```python
from build123d import *

# Parameters (mm, degrees)
CLAMP_OUTLINE_SKETCH_W = 7
CLAMP_OUTLINE_SKETCH_H = 6
CLAMP_OUTLINE_DEPTH    = 1
M2_CLEARANCE_SKETCH_R  = 1.1
M2_CLEARANCE_DEPTH     = 1.2


with BuildPart() as part:
    # Clamp Outline Sketch → Clamp Outline (new body)
    with BuildSketch(Plane.XY):
        Rectangle(CLAMP_OUTLINE_SKETCH_W, CLAMP_OUTLINE_SKETCH_H)
    extrude(amount=CLAMP_OUTLINE_DEPTH)

    # M2 Clearance Sketch → M2 Clearance (cut)
    with BuildSketch(Plane.XY.offset(-0.1)):
        Circle(M2_CLEARANCE_SKETCH_R)
    extrude(amount=M2_CLEARANCE_DEPTH, mode=Mode.SUBTRACT)


solid = part.part
```
Build history of the part. All positions in model axes, mm. Round coordinates to 2 decimals unless told otherwise and drop trailing zeros. Write each loop counter-clockwise with the first axis right and the second up, starting at its lowest first coordinate (ties: lowest second). Pieces come first, ordered by that corner, then holes.
1) Drill centre lines: probe 1 along X at (y, z) = (0, 0.4); probe 2 along Y at (x, z) = (0, 0.6); probe 3 along Y at (x, z) = (0.5, 0.2). Where is each one in solid material? Low to high.
2) Mould opens along Y. For faces 1 (the flat face through (3.5, 0, 0.5)), 2 (the flat face through (0, 3, 0.5)), 3 (the cylindrical face through (1.05, 0.33, 0.49)), 4 (the flat face through (0, -3, 0.5)) say: +Y half, -Y half, draft (parallel to the pull), parting line (faces both ways), or undercut.
3) Band-saw the part on C-C, the plane z = 0.35. List the corners of the cut face in (x, y).
4) Band-saw the part on A-A, the plane y = 0. List the corners of the cut face in (x, z).
5) Band-saw the part on B-B, the plane x = 0. List the corners of the cut face in (y, z), and give its area (3 significant figures).
Ans:
1. probe 1: x = -3.5 to -1.1, 1.1 to 3.5
1. probe 2: y = -3 to -1.1, 1.1 to 3
1. probe 3: y = -3 to -0.98, 0.98 to 3
2. face 1: draft
2. face 2: +Y half
2. face 3: undercut
2. face 4: -Y half
3. outline: (-3.5, -3) - (3.5, -3) - (3.5, 3) - (-3.5, 3) - close; hole circle Ø2.2 at (0, 0)
4. outline: (-3.5, 0) - (-1.1, 0) - (-1.1, 1) - (-3.5, 1) - close; (1.1, 0) - (3.5, 0) - (3.5, 1) - (1.1, 1) - close
5. outline: (-3, 0) - (-1.1, 0) - (-1.1, 1) - (-3, 1) - close; (1.1, 0) - (3, 0) - (3, 1) - (1.1, 1) - close
5. area: 3.80 mm2
